Source: CAD feature listing. Evaluate the final solid. Frame: model axes, mm. Round coordinates to 2 decimals unless told otherwise and drop trailing zeros. Write each loop counter-clockwise with the first axis right and the second up, starting at its lowest first coordinate (ties: lowest second). Pieces come first, ordered by that corner, then holes.
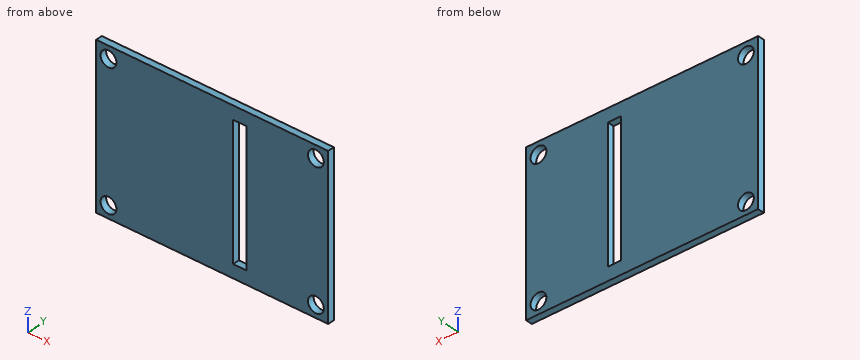
from build123d import *

# Parameters (mm, degrees)
SKETCH1_W           = 69.85
SKETCH1_H           = 48.1
SKETCH1_W_2         = 4
SKETCH1_H_2         = 40.1
BOSS_EXTRUDE1_DEPTH = 2
SKETCH2_R           = 2.38125
CUT_EXTRUDE1_DEPTH  = 2
SKETCH3_R           = 2.38125
CUT_EXTRUDE2_DEPTH  = 2
SKETCH4_R           = 2.38125
CUT_EXTRUDE3_DEPTH  = 2
SKETCH5_R           = 2.38125
CUT_EXTRUDE4_DEPTH  = 2


with BuildPart() as part:
    # Sketch1 → Boss-Extrude1 (new body)
    with BuildSketch(Plane(origin=(0, 0, 0), x_dir=(1, 0, 0), z_dir=(0, 1, 0))):
        with Locations((0.741612582, -9.055777885)):
            Rectangle(SKETCH1_W, SKETCH1_H)
        with Locations((9.056612582, -9.055777885)):
            Rectangle(SKETCH1_W_2, SKETCH1_H_2, mode=Mode.SUBTRACT)
    extrude(amount=BOSS_EXTRUDE1_DEPTH)

    # Sketch2 → Cut-Extrude1 (cut)
    with BuildSketch(Plane(origin=(0, 2, 0), x_dir=(1, 0, 0), z_dir=(0, 1, 0))):
        with Locations(Location((-30.483387418, -29.405777885, 0), (0, 0, 270))):
            Circle(SKETCH2_R)
    extrude(amount=-CUT_EXTRUDE1_DEPTH, mode=Mode.SUBTRACT)

    # Sketch3 → Cut-Extrude2 (cut)
    with BuildSketch(Plane(origin=(0, 2, 0), x_dir=(1, 0, 0), z_dir=(0, 1, 0))):
        with Locations(Location((-30.483387418, 11.294222115, 0), (0, 0, 270))):
            Circle(SKETCH3_R)
    extrude(amount=-CUT_EXTRUDE2_DEPTH, mode=Mode.SUBTRACT)

    # Sketch4 → Cut-Extrude3 (cut)
    with BuildSketch(Plane(origin=(0, 2, 0), x_dir=(1, 0, 0), z_dir=(0, 1, 0))):
        with Locations(Location((31.966612582, -29.405777885, 0), (0, 0, 270))):
            Circle(SKETCH4_R)
    extrude(amount=-CUT_EXTRUDE3_DEPTH, mode=Mode.SUBTRACT)

    # Sketch5 → Cut-Extrude4 (cut)
    with BuildSketch(Plane(origin=(0, 2, 0), x_dir=(1, 0, 0), z_dir=(0, 1, 0))):
        with Locations(Location((31.966612582, 11.294222115, 0), (0, 0, 270))):
            Circle(SKETCH5_R)
    extrude(amount=-CUT_EXTRUDE4_DEPTH, mode=Mode.SUBTRACT)


solid = part.part
1) Material intervals for line 1 (X direction, y = 1.6, z = 10.5); line 2 (Z direction, x = 31.5, y = 1.7); line 3 (Z direction, x = -28.5, y = 1), sorted ascending.
Taken from the geometry:
line 1: x = -34.18 to 7.06, 11.06 to 35.67
line 2: z = -14.99 to -13.63, -8.96 to 27.07, 31.74 to 33.11
line 3: z = -14.99 to -12.61, -9.98 to 28.09, 30.72 to 33.11
2) Section query C-C on z = -10. Return the cut outline in (x, y).
Taken from the geometry:
outline: (-34.18, 0) - (-32.48, 0) - (-32.48, 2) - (-34.18, 2) - close; (-28.48, 0) - (7.06, 0) - (7.06, 2) - (-28.48, 2) - close; (11.06, 0) - (29.97, 0) - (29.97, 2) - (11.06, 2) - close; (33.97, 0) - (35.67, 0) - (35.67, 2) - (33.97, 2) - close
3) Section query B-B on y = 0.6. Return the cut outline in (x, z).
Taken from the geometry:
outline: (-34.18, -14.99) - (35.67, -14.99) - (35.67, 33.11) - (-34.18, 33.11) - close; hole circle Ø4.76 at (-30.48, -11.29); hole circle Ø4.76 at (-30.48, 29.41); hole (7.06, -10.99) - (11.06, -10.99) - (11.06, 29.11) - (7.06, 29.11) - close; hole circle Ø4.76 at (31.97, -11.29); hole circle Ø4.76 at (31.97, 29.41)
4) Section query A-A on z = 0. Return the cut outline in (x, y), then the cut area to 3 significant figures.
Taken from the geometry:
outline: (-34.18, 0) - (7.06, 0) - (7.06, 2) - (-34.18, 2) - close; (11.06, 0) - (35.67, 0) - (35.67, 2) - (11.06, 2) - close
area: 132 mm2
